Autodesk Inventor part; units mm, degrees
ref_plane "YZ Plane" through (0, 0, 0) normal (1, 0, 0) x (0, 1, 0)
ref_plane "XZ Plane" through (0, 0, 0) normal (0, 1, 0) x (-1, 0, 0)
ref_plane "XY Plane" through (0, 0, 0) normal (0, 0, 1) x (1, 0, 0)
sketch "Sketch1" plane through (0, 0, 0) normal (0, 0, 1) x (1, 0, 0)
  line L0 (-25.4, 12.7) -> (25.4, 12.7)
  line L1 (25.4, 12.7) -> (25.4, -12.7)
  line L2 (25.4, -12.7) -> (-25.4, -12.7)
  line L3 (-25.4, -12.7) -> (-25.4, 12.7)
  line L4 (-25.4, 12.7) -> (25.4, -12.7) construction
  line L5 (25.4, 12.7) -> (-25.4, -12.7) construction
  line L6 (22.225, 9.525) -> (-22.225, 9.525)
  line L7 (-22.225, 9.525) -> (-22.225, -9.525)
  line L8 (-22.225, -9.525) -> (22.225, -9.525)
  line L9 (22.225, -9.525) -> (22.225, 9.525)
  line L10 (22.225, 9.525) -> (-22.225, -9.525) construction
  line L11 (-22.225, 9.525) -> (22.225, -9.525) construction
  point P0 (0, 0)
  dimension "d0" = 50.8
  dimension "d1" = 25.4
  dimension "d2" = 3.175
  dimension "d3" = 3.175
extrude "Extrusion1" add sketch "Sketch1" along normal mid plane 304.8
sketch "Sketch2" plane through (-25.4, 12.7, 152.4) normal (0, 1, 0) x (1, 0, 0)
  line L0 (50.8, 0) -> (0, 0)
  line L1 (0, 304.8) -> (50.8, 304.8)
  line L2 (0, 304.8) -> (0, 0)
  line L3 (50.8, 304.8) -> (50.8, 0)
  point P0 (25.4, 152.4)
  point P1 (12.7, 6.35)
  point P2 (38.1, 6.35)
  point P3 (38.1, 44.45)
  point P4 (12.7, 44.45)
  point P5 (12.7, 298.45)
  point P6 (38.1, 298.45)
  point P7 (38.1, 260.35)
  point P8 (12.7, 260.35)
  dimension "d6" = 6.35
  dimension "d7" = 25.4
  dimension "d8" = 38.1
  dimension "d9" = 6.35
  dimension "d10" = 12.7
  dimension "d11" = 12.7
  dimension "d12" = 12.7
  dimension "d13" = 38.1
hole "Hole1" at (-12.7, 12.7, 146.05) at (12.7, 12.7, 146.05) at (12.7, 12.7, 107.95) at (-12.7, 12.7, 107.95) at (-12.7, 12.7, -146.05) at (12.7, 12.7, -146.05) at (12.7, 12.7, -107.95) at (-12.7, 12.7, -107.95) direction (0, -1, 0) diameter 5.1054 end through all
properties part number "GP1-003" material "Aluminum 6061"
Build history of the part. All positions in model axes, mm. A direction names the side the tool comes from. Round coordinates to 2 decimals unless told otherwise and drop trailing zeros. Write each loop counter-clockwise with the first axis right and the second up, starting at its lowest first coordinate (ties: lowest second). Pieces come first, ordered by that corner, then holes. Notation, with made-up numbers: (77, -16) - (134, -16) arc R23 cw to (134, 10) - close; hole circle Ø4 at (-7, 46.5). An arc over 180 degrees is marked (long way). One line per question, with ' | ' between items.
1. Mould opens along Y. For faces 3 (the face through (22.225, 0, -2)), 4 (the face through (-13.467, -11.135, -143.615)), 5 (the face through (0, 12.7, -2)) say: released by +Y, released by -Y, zero draft, split by the parting line, or undercut.
Results are:
face 3: undercut | face 4: zero draft | face 5: released by +Y
2. Tool access for faces 1 (the face through (-22.225, 0, -2)), 2 (the face through (-13.467, 11.09, -143.615)): list every direction of +Z, -Z, +X, -X, +Y, -Y with a clear straight run to the whole face (end or side of a thin tool).
Results are:
face 1: +Z, -Z | face 2: +Y, -Y
3. Drop a flat-ended pin along its axis: pin 1 Ø4 at (x, z) = (12.7, 146.05) entering from +Y. Give the stop position or say it passes through.
Results are:
pin 1: through
4. Band-saw the part on B-B, the plane z = 146.05. Write the cut outline in (x, y) (3 decimals), and give its area (3 significant figures).
Results are:
outline: (-25.4, -12.7) - (-15.253, -12.7) - (-15.253, -9.525) - (-22.225, -9.525) - (-22.225, 9.525) - (-15.253, 9.525) - (-15.253, 12.7) - (-25.4, 12.7) - close; (-10.147, -12.7) - (10.147, -12.7) - (10.147, -9.525) - (-10.147, -9.525) - close; (-10.147, 9.525) - (10.147, 9.525) - (10.147, 12.7) - (-10.147, 12.7) - close; (15.253, -12.7) - (25.4, -12.7) - (25.4, 12.7) - (15.253, 12.7) - (15.253, 9.525) - (22.225, 9.525) - (22.225, -9.525) - (15.253, -9.525) - close | area: 379 mm^2
5. Band-saw the part on A-A, the plane y = -6.75. Write the cut outline in (x, z) (3 decimals).
Results are:
outline: (-25.4, -152.4) - (-22.225, -152.4) - (-22.225, 152.4) - (-25.4, 152.4) - close; (22.225, -152.4) - (25.4, -152.4) - (25.4, 152.4) - (22.225, 152.4) - close
6. Band-saw the part on C-C, the plane x = 12.7. Give the number of separate pieces and of enclosed holes in the cut face, and give its area (3 significant figures).
Results are:
separate pieces: 10 | enclosed holes: 0 | area: 1,810 mm^2
7. Drill centre lines: line 1 along Z through (x, y) = (-12.7, -10.8); line 2 along X through (y, z) = (-4.75, -73) (3 decimals); line 3 along Y through (x, z) = (1, -9) (3 decimals). Where is each one in solid material? Low to high. Write a range as from..to.
Results are:
line 1: -152.4..-148.6, -143.5..-110.5, -105.4..105.4, 110.5..143.5, 148.6..152.4 | line 2: -25.4..-22.225, 22.225..25.4 | line 3: -12.7..-9.525, 9.525..12.7
